Source: CAD feature listing. Evaluate the final solid. Frame: model axes, mm. Face numbers are marked on the shaded views. A direction names the side the tool comes from. Coordinates: 2 decimals unless noted, no trailing zeros. Loops run counter-clockwise (first coordinate to the right, second up) from the corner with the lowest first, then second, coordinate; pieces in that order, holes last. Notation, with made-up numbers: (3.5, 18.5) - (27.5, 18.5) arc R24 ccw to (27.5, 28.5) - close; hole circle Ø2 at (30.25, 89). An arc over 180 degrees is marked (long way). Write item = value, one per line. Start each with the question number.
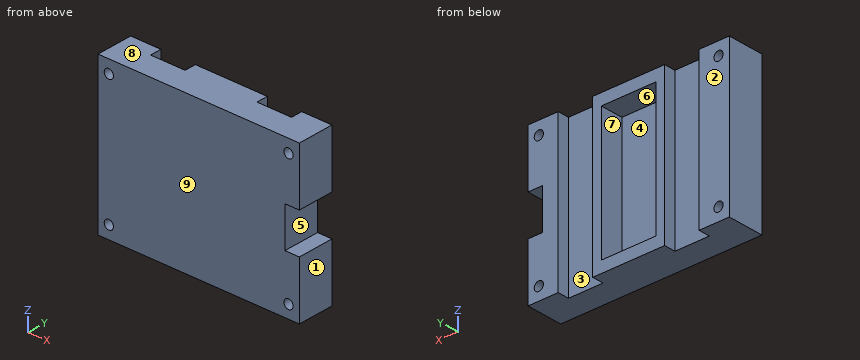
from build123d import *

# Parameters (mm, degrees)
RESSALTO_EXTRUS_O1_DEPTH   = 98
ESBO_O4_W                  = 33
ESBO_O4_H                  = 22
CORTE_EXTRUS_O3_DEPTH      = 25
ESBO_O10_W                 = 12
ESBO_O10_H                 = 4
CORTE_EXTRUS_O8_DEPTH      = 122.545423608
ESBO_O11_R                 = 1.6
CORTE_EXTRUS_O9_DEPTH      = 20
ESBO_O15_W                 = 4
ESBO_O15_H                 = 22
CORTE_EXTRUS_O11_DEPTH     = 137.386546257
CORTE_EXTRUS_O12_START     = -12.7
CORTE_EXTRUS_O12_OUTLINE_W = 5
CORTE_EXTRUS_O12_OUTLINE_H = 14
CORTE_EXTRUS_O12_DEPTH     = 12.7
ESBO_O17_W                 = 11.435879356
ESBO_O17_H                 = 99.573316557
CORTE_EXTRUS_O13_DEPTH     = 20
ESBO_O18_W                 = 19
ESBO_O18_H                 = 46
CORTE_EXTRUS_O14_DEPTH     = 8


# Read off the part's stored shape, not the designer's step: Corte-extrus_o12
with BuildPart() as part:
    # Esbo_o1 → Ressalto-extrus_o1 (new body)
    with BuildSketch(Plane.XY):
        Polygon((0, 0), (94, 0), (75.862520314, 12.7), (0, 12.7), align=None)
    extrude(amount=RESSALTO_EXTRUS_O1_DEPTH)

    # Esbo_o4 → Corte-extrus_o3 (cut)
    with BuildSketch(Plane(origin=(0, 12.7, 0), x_dir=(1, 0, 0), z_dir=(0, 1, 0))):
        with Locations((16.5, -87)):
            Rectangle(ESBO_O4_W, ESBO_O4_H)
        with Locations((16.5, -11)):
            Rectangle(ESBO_O4_W, ESBO_O4_H)
        with Locations((53.5, -87)):
            Rectangle(ESBO_O4_W, ESBO_O4_H)
        with Locations((53.5, -11)):
            Rectangle(ESBO_O4_W, ESBO_O4_H)
    extrude(amount=-CORTE_EXTRUS_O3_DEPTH, mode=Mode.SUBTRACT)

    # Esbo_o10 → Corte-extrus_o8 (cut, through all)
    with BuildSketch(Plane.XY.offset(76)):
        with Locations((16.5, 10.7)):
            Rectangle(ESBO_O10_W, ESBO_O10_H)
        with Locations((53.5, 10.7)):
            Rectangle(ESBO_O10_W, ESBO_O10_H)
    extrude(amount=-CORTE_EXTRUS_O8_DEPTH, mode=Mode.SUBTRACT)

    # Esbo_o11 → Corte-extrus_o9 (cut)
    with BuildSketch(Plane(origin=(0, 12.7, 0), x_dir=(1, 0, 0), z_dir=(0, 1, 0))):
        with Locations(Location((3.75, -71.5, 0), (0, 0, 180))):
            Circle(ESBO_O11_R)
        with Locations(Location((3.75, -26.5, 0), (0, 0, 180))):
            Circle(ESBO_O11_R)
        with Locations(Location((66.25, -26.5, 0), (0, 0, 180))):
            Circle(ESBO_O11_R)
        with Locations(Location((66.25, -71.5, 0), (0, 0, 180))):
            Circle(ESBO_O11_R)
    extrude(amount=-CORTE_EXTRUS_O9_DEPTH, mode=Mode.SUBTRACT)

    # Esbo_o15 → Corte-extrus_o11 (cut, through all)
    with BuildSketch(Plane(origin=(0, 12.7, 0), x_dir=(1, 0, 0), z_dir=(0, 1, 0))):
        with Locations((35, -11)):
            Rectangle(ESBO_O15_W, ESBO_O15_H)
        with Locations((35, -87)):
            Rectangle(ESBO_O15_W, ESBO_O15_H)
    extrude(amount=-CORTE_EXTRUS_O11_DEPTH, mode=Mode.SUBTRACT)

    # Corte-extrus_o12 outline → Corte-extrus_o12 (cut)
    with BuildSketch(Plane(origin=(0, 12.7, 0), x_dir=(1, 0, 0), z_dir=(0, 1, 0)).offset(CORTE_EXTRUS_O12_START)):
        Polygon((95.832875802, -109.85505817), (95.832875802, 2.472968948), (70, 2.472968948), (70, 0), (75.862520314, 0), (75.862520314, -98), (70, -98), (70, -109.85505817), align=None)
        with Locations((67.5, -49)):
            Rectangle(CORTE_EXTRUS_O12_OUTLINE_W, CORTE_EXTRUS_O12_OUTLINE_H)
    extrude(amount=CORTE_EXTRUS_O12_DEPTH, mode=Mode.SUBTRACT)

    # Esbo_o17 → Corte-extrus_o13 (cut)
    with BuildSketch(Plane(origin=(0, 12.7, 0), x_dir=(1, 0, 0), z_dir=(0, 1, 0))):
        with Locations((75.717939678, -49.786658279)):
            Rectangle(ESBO_O17_W, ESBO_O17_H)
    extrude(amount=-CORTE_EXTRUS_O13_DEPTH, mode=Mode.SUBTRACT)

    # Esbo_o18 → Corte-extrus_o14 (cut)
    with BuildSketch(Plane(origin=(0, 12.7, 0), x_dir=(1, 0, 0), z_dir=(0, 1, 0))):
        with Locations((35, -49)):
            Rectangle(ESBO_O18_W, ESBO_O18_H)
    extrude(amount=-CORTE_EXTRUS_O14_DEPTH, mode=Mode.SUBTRACT)


solid = part.part
Item 1: Cut plane C-C (z = 38.5). Return the cut outline in (x, y).
Item 2: Reachability of the marked faces 1, 2, 3, 4 and 5 from +Z, -Z, +X, -X, +Y, -Y: full face, straight path, thin tool, end or side. Return the list, or none.
Item 3: Cut plane A-A (x = 66.25). Return the cut outline in (y, z).
Item 4: Cut plane D-D (x = 41.5). Return the cut outline in (y, z).
Item 5: Material intervals for L1, parallel to X at y = 6.5, z = 71.5; L2, parallel to Z at x = 3.75, y = 10; L3, parallel to Z at x = 66.25, y = 4.5, sorted ascending. Write a range as [from, to].
Item 6: Draft query along Z for the marked faces 6, 7, 8 and 9. Return one class per face: released by +Z, released by -Z, zero draft, split by the parting line, or undercut.
Item 7: Cut plane B-B (y = 10.25). Return the cut outline in (x, z).
Item 8: First-contact query: pin 1 (2 mm diameter, centred on y = 11, z = 51, fed in from +X); pin 2 (1.5 mm diameter, centred on x = 19, z = 63, fed in from -Y); pin 3 (2.5 mm diameter, centred on x = 3.75, z = 71.5, fed in from +Y); pin 4 (8 mm diameter, centred on x = 18, z = 66.5, fed in from +Y). Flat tips, straight axial feed; report the tip coordinate or a pass-through.
Responses:
q1.outline = (0, 0) - (70, 0) - (70, 12.7) - (59.5, 12.7) - (59.5, 8.7) - (47.5, 8.7) - (47.5, 12.7) - (44.5, 12.7) - (44.5, 4.7) - (25.5, 4.7) - (25.5, 12.7) - (22.5, 12.7) - (22.5, 8.7) - (10.5, 8.7) - (10.5, 12.7) - (0, 12.7) - close
q2.face_1 = +Z, -Z, +X, +Y, -Y
q2.face_2 = +Z, -Z, +X, -X, +Y
q2.face_3 = +Z, -Z, +Y
q2.face_4 = +Y
q2.face_5 = +X, +Y, -Y
q3.outline = (0, 22) - (12.7, 22) - (12.7, 24.9) - (0, 24.9) - close; (0, 28.1) - (12.7, 28.1) - (12.7, 42) - (0, 42) - close; (0, 56) - (12.7, 56) - (12.7, 69.9) - (0, 69.9) - close; (0, 73.1) - (12.7, 73.1) - (12.7, 76) - (0, 76) - close
q4.outline = (0, 22) - (12.7, 22) - (12.7, 26) - (4.7, 26) - (4.7, 72) - (12.7, 72) - (12.7, 76) - (0, 76) - close
q5.L1 = [0, 2.15], [5.35, 25.5], [44.5, 64.65], [67.85, 70]
q5.L2 = [22, 24.9], [28.1, 69.9], [73.1, 76]
q5.L3 = [22, 24.9], [28.1, 42], [56, 69.9], [73.1, 76]
q6.face_6 = undercut
q6.face_7 = undercut
q6.face_8 = released by +Z
q6.face_9 = zero draft
q7.outline = (0, 22) - (10.5, 22) - (10.5, 76) - (0, 76) - close; (22.5, 22) - (47.5, 22) - (47.5, 76) - (22.5, 76) - close; (59.5, 22) - (70, 22) - (70, 42) - (65, 42) - (65, 56) - (70, 56) - (70, 76) - (59.5, 76) - close; hole circle Ø3.2 at (3.75, 26.5); hole circle Ø3.2 at (3.75, 71.5); hole (25.5, 26) - (44.5, 26) - (44.5, 72) - (25.5, 72) - close; hole circle Ø3.2 at (66.25, 26.5); hole circle Ø3.2 at (66.25, 71.5)
q8.pin_1 = 65
q8.pin_2 = 0
q8.pin_3 = through
q8.pin_4 = 8.7
